```python
from build123d import *

# Parameters (mm, degrees)
F0_W      = 25
F0_H      = 115
F1_DEPTH  = 5
F2_W      = 25
F2_H      = 5
F3_DEPTH  = 140
F4_W      = 5
F4_H      = 25
F5_DEPTH  = 110
F6_W      = 25
F6_H      = 5
F7_DEPTH  = 40
F8_W      = 25
F8_H      = 5
F9_DEPTH  = 40
F10_W     = 5
F10_H     = 105
F11_DEPTH = 20
F12_W     = 5
F12_H     = 105
F13_DEPTH = 20
F14_W     = 5
F14_H     = 20
F15_DEPTH = 97.6
F17_R     = 4
F18_DEPTH = 25
F19_R     = 4
F20_DEPTH = 15
F21_DEPTH = 25
F22_DEPTH = 25


with BuildPart() as f1:
    # F0 (on Right) → F1 (new body)
    with BuildSketch(Plane.YZ):
        Rectangle(F0_W, F0_H)
    extrude(amount=F1_DEPTH)

    # F2 (on face) → F3 (join)
    with BuildSketch(Plane(origin=(0, 0, 0), x_dir=(0, -1, 0), z_dir=(-1, 0, 0))):
        with Locations((0, 55)):
            Rectangle(F2_W, F2_H)
    extrude(amount=F3_DEPTH)

    # F4 (on face) → F5 (join)
    with BuildSketch(Plane(origin=(0, 0, 52.5), x_dir=(1, 0, 0), z_dir=(0, 0, -1))):
        with Locations((-137.5, 0)):
            Rectangle(F4_W, F4_H)
    extrude(amount=F5_DEPTH)

    # F6 (on face) → F7 (join)
    with BuildSketch(Plane.YZ.offset(-135)):
        with Locations((0, -55)):
            Rectangle(F6_W, F6_H)
    extrude(amount=F7_DEPTH)

    # F8 (on face) → F9 (join)
    with BuildSketch(Plane(origin=(0, 0, 0), x_dir=(0, -1, 0), z_dir=(-1, 0, 0))):
        with Locations((0, -55)):
            Rectangle(F8_W, F8_H)
    extrude(amount=F9_DEPTH)

    # F10 (on face) → F11 (join)
    with BuildSketch(Plane.YZ.offset(-135)):
        with Locations((10, 0)):
            Rectangle(F10_W, F10_H)
    extrude(amount=F11_DEPTH)

    # F12 (on face) → F13 (join)
    with BuildSketch(Plane(origin=(0, 0, 0), x_dir=(0, -1, 0), z_dir=(-1, 0, 0))):
        with Locations((-10, 0)):
            Rectangle(F12_W, F12_H)
    extrude(amount=F13_DEPTH)

    # F14 (on face) → F15 (join)
    with BuildSketch(Plane(origin=(-20, 0, 0), x_dir=(0, -1, 0), z_dir=(-1, 0, 0))):
        with Locations((-10, 42.5)):
            Rectangle(F14_W, F14_H)
    extrude(amount=F15_DEPTH)

    # F17 (on face) → F18 (cut)
    with BuildSketch(Plane.XY.offset(-52.5)):
        with Locations((-105, 0)):
            Circle(F17_R)
    extrude(amount=-F18_DEPTH, mode=Mode.SUBTRACT)

    # F19 (on face) → F20 (cut)
    with BuildSketch(Plane.XY.offset(-52.5)):
        with Locations((-30, 0)):
            Circle(F19_R)
    extrude(amount=-F20_DEPTH, mode=Mode.SUBTRACT)

    # F17 (on face) → F21 (cut)
    with BuildSketch(Plane.XY.offset(-52.5)):
        with Locations((-105, 0)):
            Circle(F17_R)
    extrude(amount=-F21_DEPTH, mode=Mode.SUBTRACT)

    # F19 (on face) → F22 (cut)
    with BuildSketch(Plane.XY.offset(-52.5)):
        with Locations((-30, 0)):
            Circle(F19_R)
    extrude(amount=-F22_DEPTH, mode=Mode.SUBTRACT)


solid = f1.part
```
The listing builds one solid part. Answer for the finished solid, in the listing's coordinates (mm). A direction names the side the tool comes from. Give positions to 0.01 mm unless a question says otherwise; leave off trailing zeros. Order: outer loops, then holes, each group sorted by start corner. A loop starts at its lowest first (then second) coordinate and runs counter-clockwise, first axis right, second up.
1) For faces 1 (the face through (-67, -2, 52.5)), 2 (the face through (-33.2, -2.4, -55)), 3 (the face through (-67, -12.5, 55)), 4 (the face through (-115, 10, -9)), 5 (the face through (-95, 0, -55)), determine the directions among +Z, -Z, +X, -X, +Y, -Y from which every point of the face is accessible in a straight line to the end or side of a thin tool.
Reported:
face 1: -Y
face 2: -Z
face 3: +Z, -Z, +X, -X, -Y
face 4: +Y, -Y
face 5: -Z, +Y, -Y
2) Find section B-B on y = 0. Write down the section's boundary in (x, z).
Reported:
outline: (-140, -57.5) - (-109, -57.5) - (-109, -52.5) - (-135, -52.5) - (-135, 52.5) - (0, 52.5) - (0, -52.5) - (-26, -52.5) - (-26, -57.5) - (5, -57.5) - (5, 57.5) - (-140, 57.5) - close; (-101, -57.5) - (-95, -57.5) - (-95, -52.5) - (-101, -52.5) - close; (-40, -57.5) - (-34, -57.5) - (-34, -52.5) - (-40, -52.5) - close
3) Find section A-A on z = 20.5. Write down the section's boundary in (x, y), then the cut area to 3 significant figures.
Reported:
outline: (-140, -12.5) - (-135, -12.5) - (-135, 7.5) - (-115, 7.5) - (-115, 12.5) - (-140, 12.5) - close; (-20, 7.5) - (0, 7.5) - (0, -12.5) - (5, -12.5) - (5, 12.5) - (-20, 12.5) - close
area: 450 mm2
4) Determine the mould class of faces 6 (the face through (-66, 0, 57.5)), 7 (the face through (5, 0, 1)), 8 (the face through (-67, 10, 32.5)) for opening direction Z: pulls with the +Z half, pulls with the -Z half, needs draft (parallel to the pull), parting line crosses it, or undercut.
Reported:
face 6: pulls with the +Z half
face 7: needs draft
face 8: undercut
5) Consider line 1 along Z through (x, y) = (-29.5, -4.25); line 2 along Y through (x, z) = (-30, -53.8); line 3 along X through (y, z) = (-3, 3.5). Determine where each line is inside the solid, lowest interval first.
Reported:
line 1: z = -57.5 to -52.5, 52.5 to 57.5
line 2: y = -12.5 to -4, 4 to 12.5
line 3: x = -140 to -135, 0 to 5
6) Given P1, Ø1.5, axis at x = -70, y = 1, coming from the -Z side; P2, Ø4, axis at x = -54.5, y = 11, coming from the -Z side, each flat-ended and moving along its own axis, determine where each tip first touches the part or whether it passes through.
Reported:
P1: stops at z = 52.5
P2: stops at z = 32.5
7) Find section C-C on x = -105. Write down the section's boundary in (y, z).
Reported:
outline: (-12.5, -57.5) - (-4, -57.5) - (-4, -52.5) - (-12.5, -52.5) - close; (-12.5, 52.5) - (7.5, 52.5) - (7.5, 32.5) - (12.5, 32.5) - (12.5, 57.5) - (-12.5, 57.5) - close; (4, -57.5) - (12.5, -57.5) - (12.5, -52.5) - (4, -52.5) - close
8) Find section D-D on x = -37. Write down the section's boundary in (y, z).
Reported:
outline: (-12.5, -57.5) - (12.5, -57.5) - (12.5, -52.5) - (-12.5, -52.5) - close; (-12.5, 52.5) - (7.5, 52.5) - (7.5, 32.5) - (12.5, 32.5) - (12.5, 57.5) - (-12.5, 57.5) - close
